Source: CAD feature listing. Evaluate the final solid. Frame: model axes, mm. Give positions to 0.01 mm unless a question says otherwise; leave off trailing zeros. Write each loop counter-clockwise with the first axis right and the second up, starting at its lowest first coordinate (ties: lowest second). Pieces come first, ordered by that corner, then holes.
```python
from build123d import *

# Parameters (mm, degrees)
SKETCH1_W                  = 6.35
SKETCH1_H                  = 1.5875
F_50_0_07_DIAMETER_HOLE1_D = 1.778
SCREW_PASSTHROUGHS_COUNT   = 12


with BuildPart() as part:
    # Sketch1 → Main (revolve)
    with BuildSketch(Plane.XY):
        with Locations((-41.275, 0.79375)):
            Rectangle(SKETCH1_W, SKETCH1_H)
    revolve(axis=Axis((0, 55, 0), (0, -1, 0)))

    # #50 (0.07) Diameter Hole1 (through all)
    with Locations(Plane(origin=(0, 0, 0), x_dir=(-1, 0, 0), z_dir=(0, -1, 0))):
        with Locations((41.275, 0)):
            f_50_0_07_diameter_hole1 = Hole(F_50_0_07_DIAMETER_HOLE1_D / 2)

    # Screw Passthroughs: #50 (0.07) Diameter Hole1 ×12 about axis
    screw_passthroughs_axis = Axis((0, 0, 0), (0, 1, 0))
    for i in range(1, SCREW_PASSTHROUGHS_COUNT):
        add(f_50_0_07_diameter_hole1.rotate(screw_passthroughs_axis, i * 360 / SCREW_PASSTHROUGHS_COUNT), mode=Mode.SUBTRACT)


solid = part.part
```
1. Section query C-C (y = 0.3). Give the number of separate pieces and of enclosed holes in the cut face, plus the area to 3 significant figures.
2. Section query B-B (z = 14). Return loops of the section in (x, y), plus the area to 3 significant figures.
3. Section query A-A (x = 11.5). Return loops of the section in (y, z).
4. Pin query (flat end, axial travel): P1, Ø1.1, axis at x = 35.75, z = -20.64, coming from the -Y side. Return the tip coordinate at first contact, or that it passes through.
5. Pull-direction query (X, two-part tool) for faces 1 (the cylindrical face through (-23.9, 0.8, -37.48)), 2 (the cylindrical face through (30.235, 0.805, 23.183)), 3 (the flat face through (-20, 0, -33)); classes: pulls with the +X half, pulls with the -X half, needs draft (parallel to the pull), parting line crosses it, or undercut.
6. Line query: probe 1 along X at (y, z) = (0.9, -0.5); probe 2 along X at (y, z) = (1.5, -6.5); probe 3 along Z at (x, y) = (14.5, 0.75). Output: solid intervals per line, ascending.
The answers:
1. separate pieces: 1
1. enclosed holes: 13
1. area: 1,620 mm2
2. outline: (-42.19, 0) - (-35.43, 0) - (-35.43, 1.59) - (-42.19, 1.59) - close; (35.43, 0) - (42.19, 0) - (42.19, 1.59) - (35.43, 1.59) - close
2. area: 21.4 mm2
3. outline: (0, -42.94) - (1.59, -42.94) - (1.59, -36.32) - (0, -36.32) - close; (0, 36.32) - (1.59, 36.32) - (1.59, 42.94) - (0, 42.94) - close
4. P1: passes through
5. face 1: parting line crosses it
5. face 2: undercut
5. face 3: needs draft
6. probe 1: x = -44.45 to -42.01, -40.54 to -38.1, 38.1 to 40.54, 42.01 to 44.45
6. probe 2: x = -43.97 to -37.54, 37.54 to 43.97
6. probe 3: z = -42.02 to -35.23, 35.23 to 42.02
